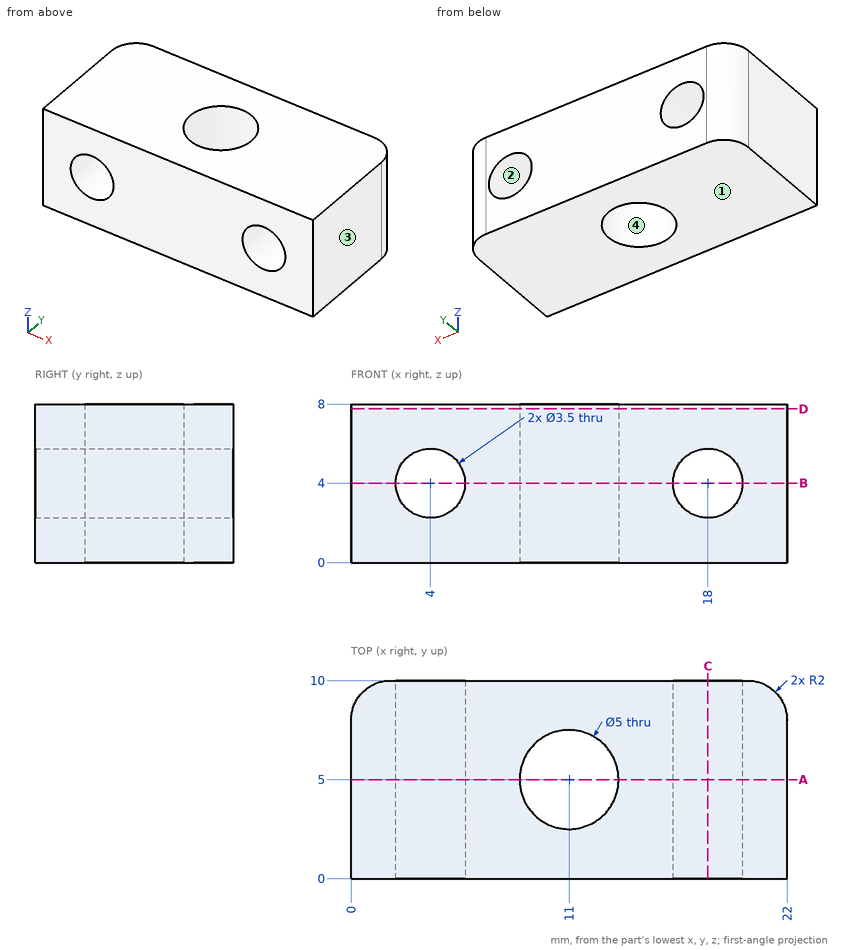
Check sheet for the drawn part. Datum: minimum x, y, z corner. Units: mm. Round coordinates to 2 decimals unless told otherwise and drop trailing zeros. Write each loop counter-clockwise with the first axis right and the second up, starting at its lowest first coordinate (ties: lowest second). Pieces come first, ordered by that corner, then holes. Notation, with made-up numbers: (46.25, 45.25) -> (69.25, 45.25) arc R9 cw to (69.25, 56.25) -> close; hole circle Ø1 at (17, 23). An arc over 180 degrees is marked (long way). One line per item, written item: value. Start each with the question number.
(1) Cross-section at A-A, the plane y = 5. Record the cut outline in (x, z), and give its area (3 significant figures).
(2) Cross-section at C-C, the plane x = 18. Record the cut outline in (y, z), and give its area (3 significant figures).
(3) Scan lines: line 1 (X direction, y = 6, z = 3.25); line 2 (X direction, y = 7.75, z = 2.75); line 3 (X direction, y = 1, z = 3.75). Record each from-to range of solid material in increasing order. Write a range as [from, to].
(4) Cross-section at D-D, the plane z = 7.75. Record the cut outline in (x, y), and give its area (3 significant figures).
(5) Cross-section at B-B, the plane z = 4. Record the cut outline in (x, y), and give its area (3 significant figures).
(6) Go/stop test with a flat-tipped pin: pin 1 Ø1.5 at (y, z) = (9, 2.5) entering from -X. Record where the tip stops, or that it passes through.
(7) Draft check along X on the marked faces 1, 2, 3 and 4. Enter one of: +X half, -X half, draft (parallel to the pull), parting line (faces both ways), or undercut.
Answer:
1. outline: (0, 0) -> (8.5, 0) -> (8.5, 8) -> (0, 8) -> close; (13.5, 0) -> (22, 0) -> (22, 8) -> (13.5, 8) -> close; hole circle Ø3.5 at (4, 4); hole circle Ø3.5 at (18, 4)
1. area: 117 mm²
2. outline: (0, 0) -> (10, 0) -> (10, 2.25) -> (0, 2.25) -> close; (0, 5.75) -> (10, 5.75) -> (10, 8) -> (0, 8) -> close
2. area: 45.0 mm²
3. line 1: [0, 2.42], [5.58, 8.71], [13.29, 16.42], [19.58, 22]
3. line 2: [0, 2.78], [5.22, 16.78], [19.22, 22]
3. line 3: [0, 2.27], [5.73, 16.27], [19.73, 22]
4. outline: (0, 0) -> (22, 0) -> (22, 8) arc R2 ccw to (20, 10) -> (2, 10) arc R2 ccw to (0, 8) -> close; hole circle Ø5 at (11, 5)
4. area: 199 mm²
5. outline: (0, 0) -> (2.25, 0) -> (2.25, 10) -> (2, 10) arc R2 ccw to (0, 8) -> close; (5.75, 0) -> (16.25, 0) -> (16.25, 10) -> (5.75, 10) -> close; (19.75, 0) -> (22, 0) -> (22, 8) arc R2 ccw to (20, 10) -> (19.75, 10) -> close; hole circle Ø5 at (11, 5)
5. area: 129 mm²
6. pin 1: x = 0.02
7. face 1: draft
7. face 2: undercut
7. face 3: +X half
7. face 4: undercut
